from build123d import *

# Parameters (mm, degrees)
F0_W     = 150
F0_H     = 75
F1_DEPTH = 3
F2_W     = 13
F2_H     = 13
F3_DEPTH = 4


with BuildPart() as f1:
    # F0 (on Front) → F1 (new body)
    with BuildSketch(Plane.XZ):
        with Locations((31.983163, 46.348685)):
            Rectangle(F0_W, F0_H)
    extrude(amount=F1_DEPTH)

    # F2 (on face) → F3 (cut)
    with BuildSketch(Plane.XZ.offset(3)):
        with Locations((-31.516837, 72.348685)):
            Rectangle(F2_W, F2_H)
        with Locations((-31.516837, 20.348685)):
            Rectangle(F2_W, F2_H)
        with Locations((95.483163, 20.348685)):
            Rectangle(F2_W, F2_H)
        with Locations((95.483163, 72.348685)):
            Rectangle(F2_W, F2_H)
        with BuildLine():
            Line((69.983163, 51.348685), (-6.016837, 51.348685))
            ThreePointArc((-6.016837, 51.348685), (-7.431051, 50.762899), (-8.016837, 49.348685))
            Line((-8.016837, 49.348685), (-8.016837, 43.348685))
            ThreePointArc((-8.016837, 43.348685), (-7.431051, 41.934472), (-6.016837, 41.348685))
            Line((-6.016837, 41.348685), (69.983163, 41.348685))
            ThreePointArc((69.983163, 41.348685), (71.397376, 41.934472), (71.983163, 43.348685))
            Line((71.983163, 43.348685), (71.983163, 49.348685))
            ThreePointArc((71.983163, 49.348685), (71.397376, 50.762899), (69.983163, 51.348685))
        make_face()
    extrude(amount=-F3_DEPTH, mode=Mode.SUBTRACT)


solid = f1.part
Read the model definition and answer for the solid it produces. Units are mm, in the model's axes. A direction names the side the tool comes from. Coordinates: 2 decimals unless noted, no trailing zeros. Loops run counter-clockwise (first coordinate to the right, second up) from the corner with the lowest first, then second, coordinate; pieces in that order, holes last. Notation, with made-up numbers: (19, -10) -> (45, -10) arc R17 cw to (45, 8) -> close; hole circle Ø6 at (36.5, 12). An arc over 180 degrees is marked (long way). Write item = value, one per line. Start each with the question number.
1) The part is cut by section D-D, the plane z = 73. Determine the outline of the cut face in (x, y).
2) For faces 3 (the face through (31, -3, 55)), 4 (the face through (-32, -2, 78.849)), determine the directions among +Z, -Z, +X, -X, +Y, -Y from which every point of the face is accessible in a straight line to the end or side of a thin tool.
3) The part is cut by section C-C, the plane z = 45.5. Determine the outline of the cut face in (x, y).
4) The mould has two halves that part along X. Classify faces 1 (the face through (31, -1, 8.849)), 2 (the face through (71.983, -2, 46)): pulls with the +X half, pulls with the -X half, needs draft (parallel to the pull), parting line crosses it, or undercut.
5) Given P1, Ø5, axis at x = 71.5, z = 39.5, coming from the +Y side, flat-ended and moving along its own axis, determine where the tip first touches the part or whether it passes through.
6) The part is cut by section B-B, the plane y = -2.4. Determine the outline of the cut face in (x, z).
7) Find the intervals of material crossed by L1, parallel to X at y = -1.7, z = 23.5; L2, parallel to Z at x = -30, y = -0.75; L3, parallel to Z at x = 41, y = -1.4, in increasing order. Write a range as from..to.
8) The part is cut by section A-A, the plane x = 49. Determine the outline of the cut face in (y, z).
Result:
q1.outline = (-43.02, -3) -> (-38.02, -3) -> (-38.02, 0) -> (-43.02, 0) -> close; (-25.02, -3) -> (88.98, -3) -> (88.98, 0) -> (-25.02, 0) -> close; (101.98, -3) -> (106.98, -3) -> (106.98, 0) -> (101.98, 0) -> close
q2.face_3 = +Z, -Z, +X, -X, -Y
q2.face_4 = +Y, -Y
q3.outline = (-43.02, -3) -> (-8.02, -3) -> (-8.02, 0) -> (-43.02, 0) -> close; (71.98, -3) -> (106.98, -3) -> (106.98, 0) -> (71.98, 0) -> close
q4.face_1 = needs draft
q4.face_2 = undercut
q5.P1 = 0
q6.outline = (-43.02, 8.85) -> (106.98, 8.85) -> (106.98, 83.85) -> (-43.02, 83.85) -> close; hole (-38.02, 13.85) -> (-25.02, 13.85) -> (-25.02, 26.85) -> (-38.02, 26.85) -> close; hole (-38.02, 65.85) -> (-25.02, 65.85) -> (-25.02, 78.85) -> (-38.02, 78.85) -> close; hole (-8.02, 43.35) arc R2 ccw to (-6.02, 41.35) -> (69.98, 41.35) arc R2 ccw to (71.98, 43.35) -> (71.98, 49.35) arc R2 ccw to (69.98, 51.35) -> (-6.02, 51.35) arc R2 ccw to (-8.02, 49.35) -> close; hole (88.98, 13.85) -> (101.98, 13.85) -> (101.98, 26.85) -> (88.98, 26.85) -> close; hole (88.98, 65.85) -> (101.98, 65.85) -> (101.98, 78.85) -> (88.98, 78.85) -> close
q7.L1 = -43.02..-38.02, -25.02..88.98, 101.98..106.98
q7.L2 = 8.85..13.85, 26.85..65.85, 78.85..83.85
q7.L3 = 8.85..41.35, 51.35..83.85
q8.outline = (-3, 8.85) -> (0, 8.85) -> (0, 41.35) -> (-3, 41.35) -> close; (-3, 51.35) -> (0, 51.35) -> (0, 83.85) -> (-3, 83.85) -> close
